Can you work these out from the drawing? Everything is in mm from the part's minimum corner. A direction names the side the tool comes from. Give positions to 0.01 mm unless a question says otherwise; leave off trailing zeros. Write each loop counter-clockwise with the first axis right and the second up, starting at its lowest first coordinate (ties: lowest second). Pieces come first, ordered by that corner, then holes. Notation, with made-up numbers: (56.5, 32.25) - (77.5, 32.25) arc R17 cw to (77.5, 50.25) - close; hole circle Ø3 at (-28, -0.5). An arc over 180 degrees is marked (long way). Use a Markdown table: item, result. Add a question column.
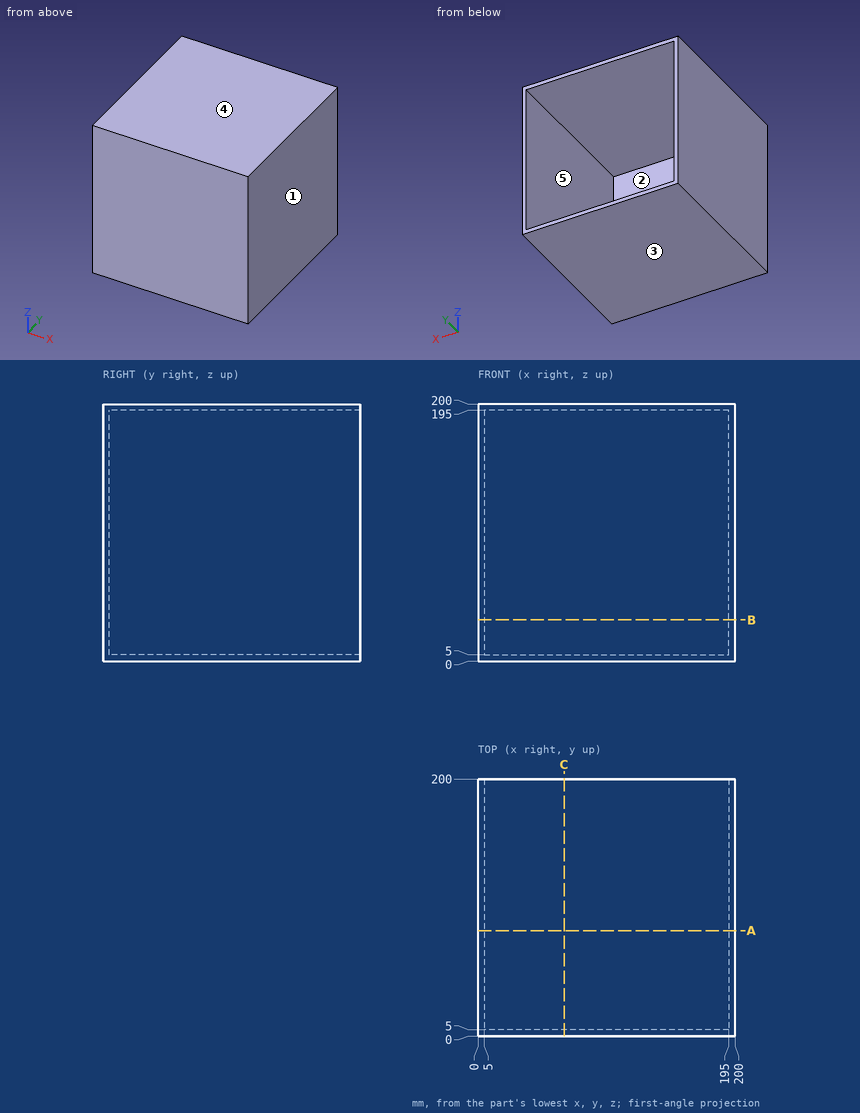
Q1. Suppose I cut it at C-C (x = 67). Please give me the cut outline in (y, z), and give its area (3 significant figures).
Q2. I'm going to push a flat-ended pin straight in: P1, Ø3, axis at x = 28, z = 75.5, coming from the +Y side. Where does the tip first touch, or does it pass through?
Q3. Suppose I cut it at A-A (y = 82). Please give me the cut outline in (x, z).
Q4. Suppose I cut it at B-B (z = 32). Please give me the cut outline in (x, y), and give its area (3 significant figures).
Q5. If we mould it in two halves opening along Z, with no side actions, what happens to the marked faces 1, 2 and 3? For each: released by +Z, released by -Z, zero draft, split by the parting line, or undercut.
Q6. If I drill on probe 1 along Z at (x, y) = (81, 114.5); probe 2 along Y at (x, z) = (80.5, 47), over which ranges is the centre line in solid material (lowest first)? Write a range as [from, to].
Q7. On a 3-axis mill with a long thin cutter (end or side, diameter ignored), from which of +Z, -Z, +X, -X, +Y, -Y can I reach the whole of each face in a straight line? I mean the marked faces 4 and 5. Say none if no direction works.
Derived:
| question | item | result |
|---|---|---|
| 1 | outline | (0, 0) - (200, 0) - (200, 5) - (5, 5) - (5, 195) - (200, 195) - (200, 200) - (0, 200) - close |
| 1 | area | 2,950 mm² |
| 2 | P1 | y = 5 |
| 3 | outline | (0, 0) - (200, 0) - (200, 200) - (0, 200) - close; hole (5, 5) - (195, 5) - (195, 195) - (5, 195) - close |
| 4 | outline | (0, 0) - (200, 0) - (200, 200) - (195, 200) - (195, 5) - (5, 5) - (5, 200) - (0, 200) - close |
| 4 | area | 2,950 mm² |
| 5 | face 1 | zero draft |
| 5 | face 2 | undercut |
| 5 | face 3 | released by -Z |
| 6 | probe 1 | [0, 5], [195, 200] |
| 6 | probe 2 | [0, 5] |
| 7 | face 4 | +Z, +X, -X, +Y, -Y |
| 7 | face 5 | +Y |
